```python
from build123d import *

# Parameters (mm, degrees)
F0_W     = 40
F0_H     = 60
F1_DEPTH = 50
F4_W     = 12
F4_H     = 7
F5_DEPTH = 50.0010001
F6_W     = 40
F6_H     = 15
F7_DEPTH = 10
F9_DEPTH = 15


with BuildPart() as f1:
    # F0 (on Front) → F1 (new body)
    with BuildSketch(Plane.XZ):
        with Locations((20, 30)):
            Rectangle(F0_W, F0_H)
    extrude(amount=F1_DEPTH)

    # F2 (on face) → F3 section 0
    with BuildSketch(Plane.XY.offset(60), mode=Mode.PRIVATE) as f3_s0:
        Polygon((40, -50), (0, 0), (0, -50), align=None)
    loft([f3_s0.sketch, Vertex(0, -50, 0)], mode=Mode.SUBTRACT)

    # F4 (on face) → F5 (cut, through all)
    with BuildSketch(Plane.XZ.offset(50)):
        with Locations((14, 3.5)):
            Rectangle(F4_W, F4_H)
    extrude(amount=-F5_DEPTH, mode=Mode.SUBTRACT)

    # F6 (on face) → F7 (cut)
    with BuildSketch(Plane.XZ.offset(50)):
        with Locations((20, 37.5)):
            Rectangle(F6_W, F6_H)
    extrude(amount=-F7_DEPTH, mode=Mode.SUBTRACT)

    # F8 (on face) → F9 (cut)
    with BuildSketch(Plane.YZ.offset(40)):
        Polygon((-50, 0), (0, 60), (-10, 60), (-50, 15), align=None)
    extrude(amount=-F9_DEPTH, mode=Mode.SUBTRACT)


solid = f1.part
```
CAD build for the part. Positions are in the model's coordinates, mm. A direction names the side the tool comes from. Round coordinates to 2 decimals unless told otherwise and drop trailing zeros. Write each loop counter-clockwise with the first axis right and the second up, starting at its lowest first coordinate (ties: lowest second). Pieces come first, ordered by that corner, then holes.
Item 1: Band-saw the part on C-C on y = -28. Write the cut outline in (x, z), then the cut area to 3 significant figures.
Filled in:
outline: (0, 0) - (8, 0) - (8, 7) - (20, 7) - (20, 0) - (40, 0) - (40, 26.4) - (25, 26.4) - (25, 39.75) - (40, 39.75) - (40, 60) - (22.4, 60) - (0, 26.4) - close
area: 1,740 mm2
Item 2: Mould opens along Y. For faces 1 (the flat face through (13.334, -30.907, 42.913)), 2 (the flat face through (14, -25, 7)), 3 (the flat face through (32.605, -29.72, 37.815)), 4 (the flat face through (25, -29, 30)) say: released by +Y, released by -Y, zero draft, split by the parting line, or undercut.
Filled in:
face 1: released by -Y
face 2: zero draft
face 3: undercut
face 4: undercut
Item 3: Band-saw the part on A-A on x = 33. Write the cut outline in (y, z), then the cut area to 3 significant figures.
Filled in:
outline: (-50, 0) - (0, 0) - (0, 60) - close; (-50, 15) - (-10, 60) - (-41.25, 60) - (-50, 49.5) - (-50, 45) - (-40, 45) - (-40, 30) - (-50, 30) - close
area: 2,200 mm2
Item 4: Drop flat-ended pins along their axis: pin 1 Ø10 at (x, y) = (34.5, -44.5) entering from +Z; pin 2 Ø5 at (x, z) = (4, 42) entering from -Y; pin 3 Ø8 at (x, y) = (29, -43.5) entering from +Z; pin 4 Ø1.5 at (x, z) = (14, 40) entering from -Y. Give the stop position or say it passes through.
Filled in:
pin 1: stops at z = 60
pin 2: stops at y = -23.76
pin 3: stops at z = 58.98
pin 4: stops at y = -35.29
Item 5: Drill centre lines: L1, parallel to Z at x = 28.5, y = -43 (3 decimals); L2, parallel to X at y = -30.5, z = 5.5; L3, parallel to Y at x = 24, z = 40. Where is each one in solid material? Low to high.
Filled in:
L1: z = 0 to 8.4, 22.875 to 30, 45 to 51.15
L2: x = 0 to 8, 20 to 40
L3: y = -40 to 0
Item 6: Tool access for faces 5 (the flat face through (30, -25, 0)), 6 (the flat face through (33, -25, 30)), 7 (the flat face through (29, -40, 38)), 8 (the flat face through (24, -19, 60)), 9 (the flat face through (20, -25, 3)): list every direction of +Z, -Z, +X, -X, +Y, -Y with a clear straight run to the whole face (end or side of a thin tool).
Filled in:
face 5: -Z, +X, -X, +Y, -Y
face 6: +X
face 7: +X, -X, -Y
face 8: +Z, +X, -X, +Y, -Y
face 9: -Z, +Y, -Y
Item 7: Band-saw the part on D-D on x = 5. Write the cut outline in (y, z), then the cut area to 3 significant figures.
Filled in:
outline: (-50, 0) - (0, 0) - (0, 60) - (-6.25, 60) - (-50, 7.5) - close
area: 1,850 mm2
Item 8: Band-saw the part on B-B on z = 46.5. Write the cut outline in (x, y).
Filled in:
outline: (0, -11.25) - (31, -50) - (40, -50) - (40, -22) - (25, -22) - (25, -11.25) - (40, -11.25) - (40, 0) - (0, 0) - close
